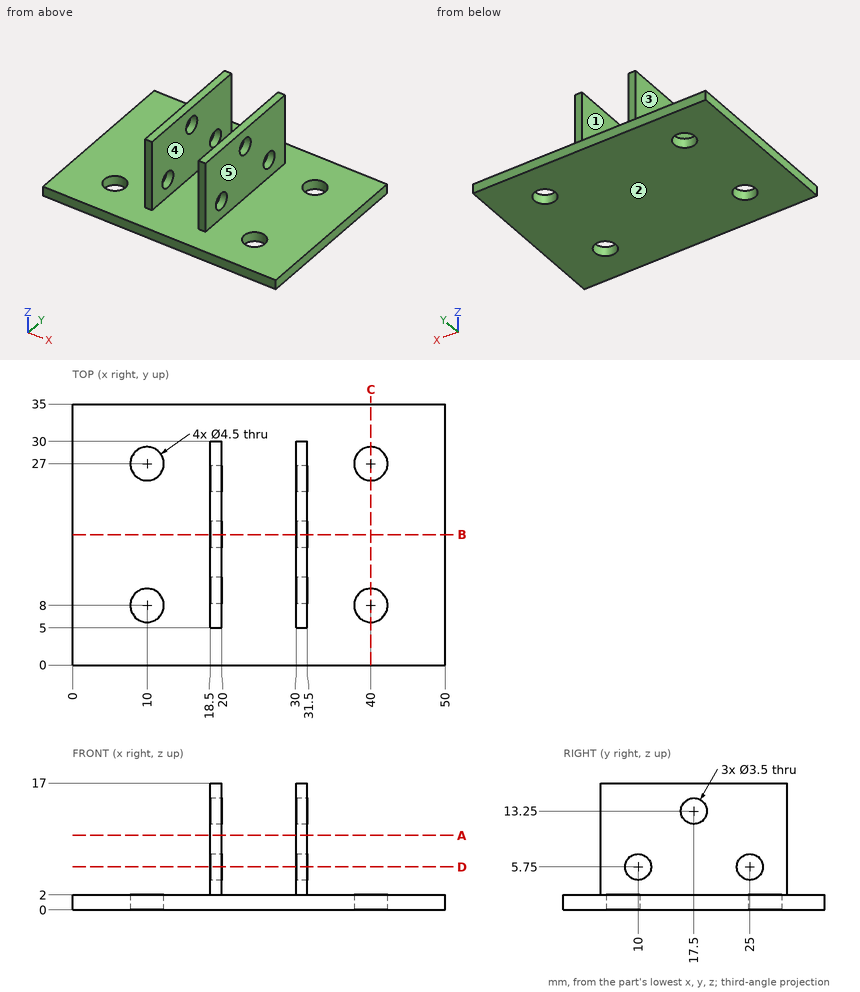
Answer from the drawing. Dimensions are ordinates in mm from the lowest x, y and z of the part. A direction names the side the tool comes from. Round coordinates to 2 decimals unless told otherwise and drop trailing zeros. Write each loop counter-clockwise with the first axis right and the second up, starting at its lowest first coordinate (ties: lowest second). Pieces come first, ordered by that corner, then holes. Notation, with made-up numbers: M 79,17.5 L 119,17.5 A29 cw 119,47.5 Z; hole C -16,31.25 d4. An arc over 180 degrees is marked long. Write each question's results on one line, items separated by ' | '. Start each with the question number.
Item 1: A cutting plane is placed at C-C on x = 40. Write down the section's boundary in (y, z).
Item 2: A cutting plane is placed at D-D on z = 5.75. Write down the section's boundary in (x, y).
Item 3: Straight lines are drawn through the part: L1, parallel to Y at x = 31, z = 5.75; L2, parallel to Y at x = 40, z = 0.4; L3, parallel to X at y = 21.5, z = 3. For each, find the intervals that lie inside material, in ascending order. Write a range as [from, to].
Item 4: A cutting plane is placed at B-B on y = 17.5. Write down the section's boundary in (x, z), and give its area (4 significant figures).
Item 5: For the marked faces 4 and 5, determine the directions among +Z, -Z, +X, -X, +Y, -Y from which every point of the face is accessible in a straight line to the end or side of a thin tool.
Item 6: A cutting plane is placed at A-A on z = 10. Write down the section's boundary in (x, y), and give its area (3 significant figures).
Item 7: For a pull along X with two mould halves and no side action, classify the marked faces 1, 2 and 3 as pulls with the +X half, pulls with the -X half, needs draft (parallel to the pull), parting line crosses it, or undercut.
Item 8: Flat-ended cylindrical pins translate along their axes: pin 1 Ø3 at (y, z) = (13, 5) entering from -X; pin 2 Ø1.5 at (x, z) = (36.5, 3) entering from -Y; pin 3 Ø0.8 at (x, z) = (19, 11) entering from -Y; pin 4 Ø5 at (y, z) = (28.5, 9.5) entering from +X. Find the tip coordinate at first contact, or state that the pin passes through.
Check sheet entries:
1) outline: M 0,0 L 5.75,0 L 5.75,2 L 0,2 Z; M 10.25,0 L 24.75,0 L 24.75,2 L 10.25,2 Z; M 29.25,0 L 35,0 L 35,2 L 29.25,2 Z
2) outline: M 18.5,5 L 20,5 L 20,8.25 L 18.5,8.25 Z; M 18.5,11.75 L 20,11.75 L 20,23.25 L 18.5,23.25 Z; M 18.5,26.75 L 20,26.75 L 20,30 L 18.5,30 Z; M 30,5 L 31.5,5 L 31.5,8.25 L 30,8.25 Z; M 30,11.75 L 31.5,11.75 L 31.5,23.25 L 30,23.25 Z; M 30,26.75 L 31.5,26.75 L 31.5,30 L 30,30 Z
3) L1: [5, 8.25], [11.75, 23.25], [26.75, 30] | L2: [0, 5.75], [10.25, 24.75], [29.25, 35] | L3: [18.5, 20], [30, 31.5]
4) outline: M 0,0 L 50,0 L 50,2 L 31.5,2 L 31.5,11.5 L 30,11.5 L 30,2 L 20,2 L 20,11.5 L 18.5,11.5 L 18.5,2 L 0,2 Z; M 18.5,15 L 20,15 L 20,17 L 18.5,17 Z; M 30,15 L 31.5,15 L 31.5,17 L 30,17 Z | area: 134.5 mm²
5) face 4: +Z, +Y, -Y | face 5: +Z, +X, +Y, -Y
6) outline: M 18.5,5 L 20,5 L 20,30 L 18.5,30 Z; M 30,5 L 31.5,5 L 31.5,30 L 30,30 Z | area: 75.0 mm²
7) face 1: undercut | face 2: needs draft | face 3: pulls with the -X half
8) pin 1: x = 18.5 | pin 2: through | pin 3: y = 5 | pin 4: x = 31.5
